Could you check a few things on this drawing? It's one solid part, dimensions in mm from its lowest x, y, z. A direction names the side the tool comes from. Give positions to 0.01 mm unless a question says otherwise; leave off trailing zeros. Loops run counter-clockwise (first coordinate to the right, second up) from the corner with the lowest first, then second, coordinate; pieces in that order, holes last. Notation, with made-up numbers: M -30,73.25 L -17,73.25 A34 cw -17,110.25 Z; hole C 31.25,73 d11. An arc over 180 degrees is marked long. Answer as a JSON object with one key per item and string values.
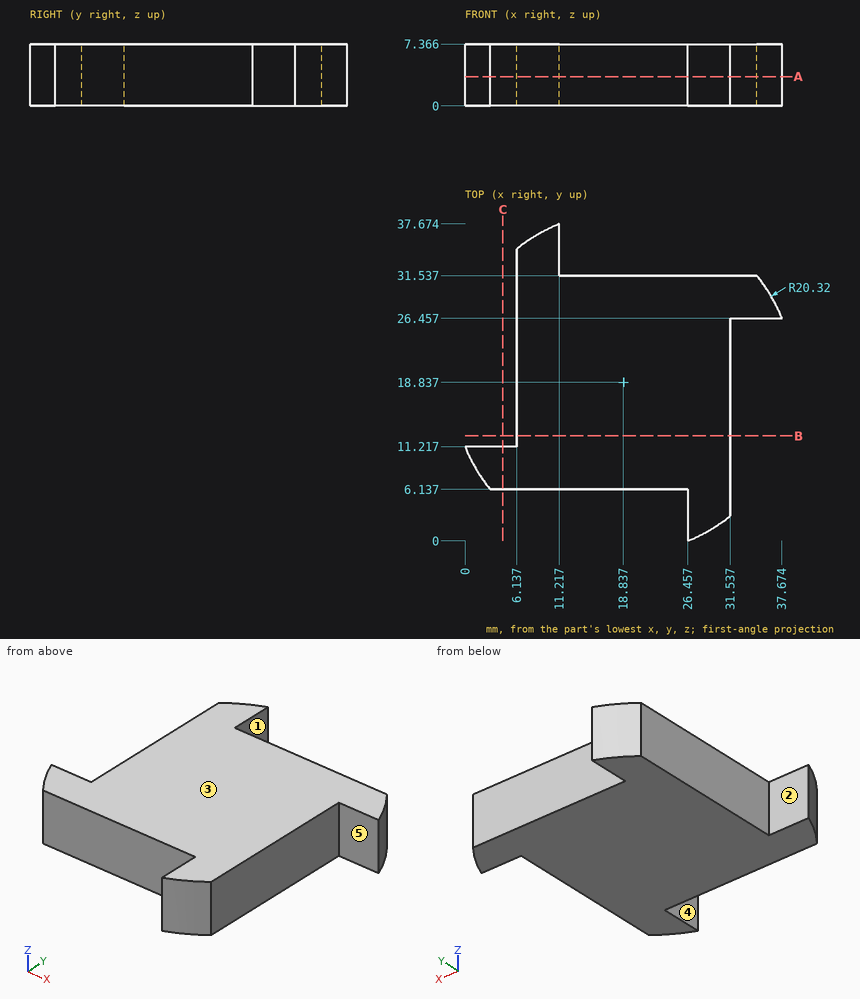
1) Suppose I cut it at C-C, the plane x = 4.5. Write out the boundary of the cut face in (y, z).
Answer list:
{"outline": "M 6.14,0 L 11.22,0 L 11.22,7.37 L 6.14,7.37 Z"}
2) For the marked faces 1, 2, 3, 4 and 5, which set-ups out of +Z, -Z, +X, -X, +Y, -Y let a thin tool reach every point of the face, with its end or its side?
Answer list:
{"face 1": "+Z, -Z, +X, +Y", "face 2": "+Z, -Z, -X, +Y", "face 3": "+Z, +X, -X, +Y, -Y", "face 4": "+Z, -Z, -X, -Y", "face 5": "+Z, -Z, +X, -Y"}
3) Suppose I cut it at B-B, the plane y = 12.5. Write out the boundary of the cut face in (x, z).
Answer list:
{"outline": "M 6.14,0 L 31.54,0 L 31.54,7.37 L 6.14,7.37 Z"}
4) Suppose I cut it at A-A, the plane z = 3.5. Write out the boundary of the cut face in (x, y) (1 decimal), and give its area (3 significant figures).
Answer list:
{"outline": "M 0,11.2 A20.3 ccw 3,6.1 L 26.5,6.1 L 26.5,0 A20.3 ccw 31.5,3 L 31.5,26.5 L 37.7,26.5 A20.3 ccw 34.7,31.5 L 11.2,31.5 L 11.2,37.7 A20.3 ccw 6.1,34.7 L 6.1,11.2 Z", "area": "743 mm^2"}
5) Will these pins go through, and if not, where does the flat tip stop? pin 1 Ø1.8 at (y, z) = (2, 4.5) entering from -X; pin 2 Ø4 at (x, z) = (13, 5) entering from -Y; pin 3 Ø1.5 at (x, z) = (23, 6) entering from +Y.
Answer list:
{"pin 1": "x = 26.46", "pin 2": "y = 6.14", "pin 3": "y = 31.54"}
6) Please list where these lines run through material, in increasing order: line 1 along Y through (x, z) = (5, 6.5); line 2 along X through (y, z) = (16, 5.75). Write a range as from..to.
Answer list:
{"line 1": "6.14..11.22", "line 2": "6.14..31.54"}
